```python
from build123d import *

# Parameters (mm, degrees)
SKETCH11_W                 = 195
SKETCH11_H                 = 100
BOSS_EXTRUDE2_DEPTH        = 15
SKETCH2_R                  = 15.5
CUT_EXTRUDE1_DEPTH         = 202.866292382
M6_TAPPED_HOLE1_D          = 5
M6_TAPPED_HOLE1_DEPTH      = 12
M6_TAPPED_HOLE1_TIP        = 1.502151548
F_6_5_6_5_DIAMETER_HOLE1_D = 6.5
M5_TAPPED_HOLE1_D          = 4.2
M5_TAPPED_HOLE1_DEPTH      = 12
M5_TAPPED_HOLE1_TIP        = 1.2618073
M6_TAPPED_HOLE2_D          = 5


with BuildPart() as part:
    # Sketch11 → Boss-Extrude2 (new body)
    with BuildSketch(Plane(origin=(0, 0, 0), x_dir=(0, 0, -1), z_dir=(1, 0, 0))):
        with Locations((-97.5, 0)):
            Rectangle(SKETCH11_W, SKETCH11_H)
    extrude(amount=-BOSS_EXTRUDE2_DEPTH)

    # Sketch2 → Cut-Extrude1 (cut, through all)
    with BuildSketch(Plane(origin=(0, 0, 0), x_dir=(0, 0, -1), z_dir=(1, 0, 0))):
        with Locations((-170, 0)):
            Circle(SKETCH2_R)
    extrude(amount=-CUT_EXTRUDE1_DEPTH, mode=Mode.SUBTRACT)

    # M6 Tapped Hole1
    with Locations(Plane(origin=(-11.981616001, -34.658638116, 0), x_dir=(-1, 0, 0), z_dir=(0, 0, -1))):
        with Locations((-4.481616001, -0.341361884), (-4.481616001, 69.658638116)):
            Hole(M6_TAPPED_HOLE1_D / 2, depth=M6_TAPPED_HOLE1_DEPTH)
            with Locations((0, 0, -(M6_TAPPED_HOLE1_DEPTH + M6_TAPPED_HOLE1_TIP / 2))):  # 118° drill point
                Cone(0, M6_TAPPED_HOLE1_D / 2, M6_TAPPED_HOLE1_TIP, mode=Mode.SUBTRACT)

    # Ø6.5 (6.5) Diameter Hole1 (through all)
    with Locations(Plane(origin=(0, -7.362824857, 24.874407607), x_dir=(0, 0, -1), z_dir=(1, 0, 0))):
        with Locations((-80.125592393, -35.137175143), (-37.625592393, -35.137175143), (4.874407607, -35.137175143), (-80.125592393, 49.862824857), (-37.625592393, 49.862824857), (4.874407607, 49.862824857)):
            Hole(F_6_5_6_5_DIAMETER_HOLE1_D / 2)

    # M5 Tapped Hole1
    with Locations(Plane(origin=(0, -36.291159976, 74.046897255), x_dir=(0, 0, 1), z_dir=(1, 0, 0))):
        with Locations((63.953102745, 7.208840024), (112.953102745, 7.208840024), (112.953102745, -79.791159976), (63.953102745, -79.791159976)):
            Hole(M5_TAPPED_HOLE1_D / 2, depth=M5_TAPPED_HOLE1_DEPTH)
            with Locations((0, 0, -(M5_TAPPED_HOLE1_DEPTH + M5_TAPPED_HOLE1_TIP / 2))):  # 118° drill point
                Cone(0, M5_TAPPED_HOLE1_D / 2, M5_TAPPED_HOLE1_TIP, mode=Mode.SUBTRACT)

    # M6 Tapped Hole2 (through all)
    with Locations(Plane(origin=(0, -42.104801514, 47.963156397), x_dir=(0, 0, -1), z_dir=(1, 0, 0))):
        with Locations((-122.036843603, 7.604801514), (-122.036843603, 76.604801514)):
            Hole(M6_TAPPED_HOLE2_D / 2)


solid = part.part
```
Geometry check sheet. Reference: the model listing, model coordinates, mm. A direction names the side the tool comes from. Coordinates: 2 decimals unless noted, no trailing zeros. Order: outer loops, then holes, each group sorted by start corner. A loop starts at its lowest first (then second) coordinate and runs counter-clockwise, first axis right, second up.
Item 1: Depth check by flat-ended pin: pin 1 (4.5 mm diameter, centred on x = -7.5, y = 35, fed in from -Z); pin 2 (4 mm diameter, centred on y = 42.5, z = 62.5, fed in from +X); pin 3 (3 mm diameter, centred on x = -7.5, y = -35, fed in from -Z). Enter the tip coordinate at first touch or a pass-through.
Item 2: Mould release check, pull along Z, two halves, no side actions. Record for faces 3 (the conical face through (-7.44, -34.57, 13.24)), 4 (the cylindrical face through (-7.605, -45.673, 19.295)), 5 (the cylindrical face through (-8.04, 32.56, 6.08)): released by +Z, released by -Z, zero draft, split by the parting line, or undercut.
Item 3: Section check A-A (x = -2.5). Count the separate pieces of the cut face and the enclosed holes in it, plus the area to 3 significant figures.
Item 4: Tool access check on faces 1 (the cylindrical face through (-7.605, 40.522, 59.921)), 2 (the cylindrical face through (-6.08, 44.3, 185.06)). Record the directions out of +Z, -Z, +X, -X, +Y, -Y that give a thin tool (end or side, any length) a straight path to the whole face; none if there is none.
Item 5: Section check B-B (z = 105). Enter the section's corners in (x, y).
Item 6: Scan lines: line 1 along Y through (x, z) = (-3.5, 62.5); line 2 along Y through (x, z) = (-5.5, 138); line 3 along Z through (x, y) = (-10.75, 44). Record each from-to range of solid material in increasing order.
Item 7: Section check C-C (z = 170). Enter the section's corners in (x, y).
Check sheet entries:
1. pin 1: stops at z = 12.15
1. pin 2: passes through
1. pin 3: stops at z = 12.6
2. face 3: released by -Z
2. face 4: undercut
2. face 5: zero draft
3. separate pieces: 1
3. enclosed holes: 13
3. area: 18,500 mm2
4. face 1: +X, -X
4. face 2: +X
5. outline: (-15, -50) - (0, -50) - (0, -45.75) - (-15, -45.75) - close; (-15, -39.25) - (0, -39.25) - (0, 39.25) - (-15, 39.25) - close; (-15, 45.75) - (0, 45.75) - (0, 50) - (-15, 50) - close
6. line 1: y = -50 to -45.75, -39.25 to 39.25, 45.75 to 50
6. line 2: y = -50 to -45.6, -41.4 to 41.4, 45.6 to 50
6. line 3: z = 0 to 17.12, 22.88 to 59.62, 65.38 to 102.12, 107.88 to 135.96, 140.04 to 184.96, 189.04 to 195
7. outline: (-15, -50) - (0, -50) - (0, -37) - (-15, -37) - close; (-15, -32) - (0, -32) - (0, -15.5) - (-15, -15.5) - close; (-15, 15.5) - (0, 15.5) - (0, 32) - (-15, 32) - close; (-15, 37) - (0, 37) - (0, 50) - (-15, 50) - close
